from build123d import *

# Parameters (mm, degrees)
F0_W     = 48
F0_H     = 12
F1_DEPTH = 60
F2_T     = -1
F3_R     = 1.5


with BuildPart() as f1:
    # F0 (on Top) → F1 (new body)
    with BuildSketch(Plane.XY):
        Rectangle(F0_W, F0_H)
    extrude(amount=F1_DEPTH)

    # F2
    f2_openings = [f1.faces().sort_by_distance(p)[0] for p in [
        (0, 6, 30),
    ]]
    offset(amount=F2_T, openings=f2_openings)

    # F3
    f3_edges = [f1.edges().sort_by_distance(p)[0] for p in [
        (24, -6, 30),
        (-24, -6, 30),
    ]]
    fillet(f3_edges, radius=F3_R)


solid = f1.part
Geometry: final body of the model. Coordinates: model frame, mm. A direction names the side the tool comes from. Round coordinates to 2 decimals unless told otherwise and drop trailing zeros. Loops run counter-clockwise (first coordinate to the right, second up) from the corner with the lowest first, then second, coordinate; pieces in that order, holes last. Notation, with made-up numbers: M -4.5,44 L 31.5,44 A30 cw 31.5,82 Z; hole C 49,17.5 d11. An arc over 180 degrees is marked long. One line per question, with ' | ' between items.
(1) Cut plane C-C on z = 41.5. Return the cut outline in (x, y).
Check result:
outline: M -24,-4.5 A1.5 ccw -22.5,-6 L 22.5,-6 A1.5 ccw 24,-4.5 L 24,6 L 23,6 L 23,-5 L -23,-5 L -23,6 L -24,6 Z
(2) Cut plane B-B on y = -2.75. Return the cut outline in (x, z), plus the area to 3 significant figures.
Check result:
outline: M -24,0 L 24,0 L 24,60 L -24,60 Z; hole M -23,1 L 23,1 L 23,59 L -23,59 Z | area: 212 mm2
(3) Material intervals for line 1 along Z through (x, y) = (17, -4.25); line 2 along X through (y, z) = (3.25, 55.5); line 3 along Y through (x, z) = (2.5, 22), sorted ascending. Write a range as from..to.
Check result:
line 1: z = 0..1, 59..60 | line 2: x = -24..-23, 23..24 | line 3: y = -6..-5
(4) Access query for faces 5 (the cylindrical face through (-23.57, -5.55, 30.42)), 6 (the flat face through (23, 0, 30)). Directions: +Z, -Z, +X, -X, +Y, -Y. A direction counts if a zero-diameter tool reaches every point of the face in a straight line with its end or side. Return the directions, or none.
Check result:
face 5: +Z, -Z, -X, -Y | face 6: +Y
(5) Pull-direction query (X, two-part tool) for faces 1 (the cylindrical face through (23.55, -5.57, 30.42)), 2 (the flat face through (0, -5, 30)), 3 (the flat face through (0, -6, 30)), 4 (the flat face through (-23, 0, 30)); classes: +X half, -X half, draft (parallel to the pull), parting line (faces both ways), or undercut.
Check result:
face 1: +X half | face 2: undercut | face 3: draft | face 4: undercut
(6) Cut plane A-A on x = 9. Return the cut outline in (y, z).
Check result:
outline: M -6,0 L 6,0 L 6,1 L -5,1 L -5,59 L 6,59 L 6,60 L -6,60 Z
